Autodesk Inventor part; units mm, degrees
ref_plane "YZ Plane" through (0, 0, 0) normal (1, 0, 0) x (0, 1, 0)
ref_plane "XZ Plane" through (0, 0, 0) normal (0, 1, 0) x (-1, 0, 0)
ref_plane "XY Plane" through (0, 0, 0) normal (0, 0, 1) x (1, 0, 0)
sketch "Эскиз1" plane through (0, 0, 0) normal (0, 1, 0) x (-1, 0, 0)
  circle A0 centre (0, 0) radius 7.95
  circle A1 centre (0, 0) radius 8.95
  line L0 (0, 0) -> (7.1419, 5.394)
  line L1 (0, 0) -> (7.1419, -5.394)
  point P0 (6.3439, -4.7913)
  point P1 (6.3439, 4.7913)
  dimension "d0" = 15.9
  dimension "d1" = 17.9
extrude "Выдавливание1" add sketch "Эскиз1" along normal blind 30 contours A0 L1 A1 L0 picked at (-8.5243, 0.7366)
sketch "Эскиз2" plane through (0, 30, 0) normal (0, 1, 0) x (1, 0, 0)
  arc A0 (-6.3439, -4.7913) -> (-7.2366, -4.2614) centre (-9.0453, -8.3253) ccw
  arc A1 (-7.2366, -4.2614) -> (-8.3936, -6.0672) centre (-7.671, -5.2567) ccw
  line L0 (-8.3936, -6.0672) -> (-7.7223, -5.2127)
  arc A2 (-7.1433, -5.3795) -> (-7.7223, -5.2127) centre (-7.5117, -5.5699) ccw
  line L1 (-6.3439, -4.7913) -> (-7.1419, -5.394)
  line L2 (-7.1419, -5.394) -> (-6.3439, -4.7913)
  line L3 (-7.1419, -5.394) -> (-7.1433, -5.3795)
  line L4 (-0.0151, 0) -> (-3.489, 0)
  arc A3 (-7.2366, 4.2614) -> (-6.3439, 4.7913) centre (-9.0453, 8.3253) ccw
  arc A4 (-7.7223, 5.2127) -> (-7.1433, 5.3795) centre (-7.5117, 5.5699) ccw
  line L5 (-6.3439, 4.7913) -> (-7.1419, 5.394)
  line L6 (-7.1419, 5.394) -> (-6.3439, 4.7913)
  line L7 (-7.1419, 5.394) -> (-7.1433, 5.3795)
  arc A5 (-8.3936, 6.0672) -> (-7.2366, 4.2614) centre (-7.671, 5.2567) ccw
  line L8 (-8.3936, 6.0672) -> (-7.7223, 5.2127)
  point P0 (-6.3439, 4.7913)
  point P1 (-7.1419, -5.394)
  point P2 (-5.3694, -4.0591)
  point P3 (-7.1419, 5.394)
  point P4 (-5.3694, 4.0591)
  point P5 (-7.1419, 5.394)
  dimension "d25" = 1.0859
sketch "Эскиз3" plane through (0, 30, 0) normal (0, 1, 0) x (1, 0, 0)
  arc A0 (-7.1419, -5.394) -> (-7.1419, 5.394) centre (0, 0) ccw
  line L0 (11.5, -6.95) -> (11.5, 6.95)
  arc A1 (-6.3439, -4.7913) -> (-6.3439, 4.7913) centre (0, 0) ccw
  arc A2 (0, -7.95) -> (0, 7.95) centre (2.8636, 0) ccw
  line L1 (0, -8.95) -> (0, -7.95)
  line L2 (0, 7.95) -> (0, 8.95)
  line L3 (11.5, 6.95) -> (11.5, 10.95)
  line L4 (11.5, -6.95) -> (11.5, -10.95)
  line L5 (0, 4.45) -> (0, 8.95)
  line L6 (11.5, -10.95) -> (0, -10.95)
  line L7 (0, -10.95) -> (0, -8.95)
  line L8 (11.5, 10.95) -> (0, 10.95)
  line L9 (0, 10.95) -> (0, 8.95)
  point P0 (0, 7.95)
  dimension "d13" = 4
  dimension "d14" = 4
  dimension "d22" = 21.9
  dimension "d23" = 3
extrude "Выдавливание3" add sketch "Эскиз3" against normal blind 30 contours L1 A2 A0 | A0 A2 L9 L8 L3 L0 L4 L6 L7 | A2 L2 A0
ref_plane "РабПлоскость1" through (11.5, 20, 4.95) normal (1, 0, 0) x (0, 0, -1)
sketch "Эскиз4" plane through (11.5, 20, 4.95) normal (1, 0, 0) x (0, 0, -1)
  line L0 (4.95, -20) -> (4.95, 10)
  line L1 (1, 10) -> (8.9, 10)
  circle A0 centre (4.95, -12) radius 5
  line L2 (14.4, -20) -> (-4.5, -20)
  circle A1 centre (4.95, 2) radius 5
  line L3 (-4.5, 10) -> (14.4, 10)
  point P0 (7.3306, 10)
  point P1 (2.5694, 10)
  point P2 (4.95, 10)
  dimension "d15" = 10
  dimension "d16" = 8
  dimension "d17" = 10
  dimension "d18" = 8
extrude "Выдавливание4" cut sketch "Эскиз4" against normal blind 2
extrude "Выдавливание5" add sketch "Эскиз2" against normal blind 30
sketch "Эскиз5" plane through (0, 30, 0) normal (0, 1, 0) x (1, 0, 0)
  arc A0 (0, 8.95) -> (-7.1419, 5.394) centre (0, 0) ccw
  line L0 (-7.1419, 5.394) -> (-7.1433, 5.3795)
  arc A1 (-7.7223, 5.2127) -> (-7.1433, 5.3795) centre (-7.5117, 5.5699) ccw
  line L1 (-7.7223, 5.2127) -> (-8.3936, 6.0672)
  arc A2 (-8.3936, 6.0672) -> (-7.2366, 4.2614) centre (-7.671, 5.2567) ccw
  arc A3 (-7.2366, 4.2614) -> (-6.3439, 4.7913) centre (-9.0453, 8.3253) ccw
  arc A4 (-6.3439, -4.7913) -> (-6.3439, 4.7913) centre (0, 0) ccw
  arc A5 (-6.3439, -4.7913) -> (-7.2366, -4.2614) centre (-9.0453, -8.3253) ccw
  arc A6 (-7.2366, -4.2614) -> (-8.3936, -6.0672) centre (-7.671, -5.2567) ccw
  line L2 (-8.3936, -6.0672) -> (-7.7223, -5.2127)
  arc A7 (-7.1433, -5.3795) -> (-7.7223, -5.2127) centre (-7.5117, -5.5699) ccw
  line L3 (-7.1433, -5.3795) -> (-7.1419, -5.394)
  arc A8 (-7.1419, -5.394) -> (0, -8.95) centre (0, 0) ccw
  line L4 (0, -8.95) -> (0, -10.95)
  line L5 (0, -10.95) -> (11.5, -10.95)
  line L6 (11.5, -10.95) -> (11.5, 10.95)
  line L7 (11.5, 10.95) -> (0, 10.95)
  line L8 (0, 10.95) -> (0, 8.95)
  arc A9 (2.9509, -8.4495) -> (2.9509, 8.4495) centre (2.8636, 0) ccw
  arc A10 (2.9509, -8.4495) -> (2.9509, 8.4495) centre (0, 0) ccw
  line L9 (0, 7.95) -> (0, 8.95)
  line L10 (0, -7.95) -> (0, -8.95)
extrude "Выдавливание6" add sketch "Эскиз5" against normal blind 30 contours A10 A9
sketch "Эскиз6" plane through (11.5, 30, 10.95) normal (1, 0, 0) x (0, 0, -1)
  circle A0 centre (10.95, -22) radius 5
  circle A1 centre (10.95, -8) radius 5
  point P0 (10.95, -30)
extrude "Выдавливание7" cut sketch "Эскиз6" against normal blind 2
properties part number "крепление маркера 16мм"
Can you work these out from the model? Positions are in its coordinate system, mm. A direction names the side the tool comes from. Coordinates: 2 decimals unless noted, no trailing zeros. Write each loop counter-clockwise with the first axis right and the second up, starting at its lowest first coordinate (ties: lowest second). Pieces come first, ordered by that corner, then holes.
Q1. Imagine slicing it at B-B, the plane x = -4.5. List the corners of the cut face in (y, z) for me, plus the area to 3 significant figures.
Results found:
outline: (0, -7.74) - (30, -7.74) - (30, -6.55) - (0, -6.55) - close; (0, 6.55) - (30, 6.55) - (30, 7.74) - (0, 7.74) - close
area: 71.0 mm2
Q2. If we mould it in two halves opening along Z, with no side actions, what happens to faces 1 (the face through (9.5, 8, 0)), 2 (the face through (-8.57, 15.21, 4.65)), 3 (the face through (-8.063, 15.21, 5.646)), 4 (the face through (-4.041, 14.79, -7.986))? For each: +Z half, -Z half, draft (parallel to the pull), parting line (faces both ways), or undercut.
Results found:
face 1: undercut
face 2: undercut
face 3: +Z half
face 4: -Z half
Q3. For P1, Ø3, axis at x = -3.5, y = 22, coming from the -Z side; P2, Ø2, axis at x = -2, y = 20, coming from the -Z side; P3, Ø2, axis at y = 10.5, z = 10.5, coming from the -X side, each with a flat end and sliding along its axis, tell me the tip position at first contact or that it passes through.
Results found:
P1: stops at z = -8.72
P2: stops at z = -8.89
P3: stops at x = 0
Q4. Imagine slicing it at D-D, the plane z = 0. List the corners of the cut face in (x, y) for me.
Results found:
outline: (7.95, 0) - (11.5, 0) - (11.5, 3) - (9.5, 3) - (9.5, 13) - (11.5, 13) - (11.5, 17) - (9.5, 17) - (9.5, 27) - (11.5, 27) - (11.5, 30) - (7.95, 30) - close
Q5. Please list where these lines run through material, in increasing order: L1, parallel to Y at x = 10.55, z = 0; L2, parallel to X at y = 5.25, z = -5.75; L3, parallel to Z at x = 11, y = 8.
Results found:
L1: y = 0 to 3, 13 to 17, 27 to 30
L2: x = -8.64 to -8.14, -6.86 to -5.49, 5.49 to 11.5
L3: z = -10.95 to -5, 5 to 10.95
Q6. Which directions (+Z, -Z, +X, -X, +Y, -Y) give clear straight access to the entire face, cutting with the end or side of a thin tool? Please do faces 5 (the face through (10.51, 17.12, 1.08)), 6 (the face through (-6.768, 15.21, 4.504)), 7 (the face through (-8.063, 15.21, -5.646)), 8 (the face through (0, 15, -10)), 9 (the face through (0, 15, 10)).
Results found:
face 5: +X
face 6: +Y, -Y
face 7: -Z, +Y, -Y
face 8: -Z, -X, +Y, -Y
face 9: +Z, -X, +Y, -Y
Q7. Imagine slicing it at C-C, the plane x = 10.5. List the corners of the cut face in (y, z) for me, plus the area to 3 significant figures.
Results found:
outline: (0, -10.95) - (30, -10.95) - (30, 10.95) - (0, 10.95) - close; hole circle Ø10 at (8, 0); hole circle Ø10 at (22, 0)
area: 500 mm2
Q8. Imagine slicing it at A-A, the plane z = -6.5. List the corners of the cut face in (x, y) for me, plus the area to 3 significant figures.
Results found:
outline: (-6.15, 0) - (-4.58, 0) - (-4.58, 30) - (-6.15, 30) - close; (4.58, 0) - (11.5, 0) - (11.5, 30) - (4.58, 30) - close
area: 255 mm2
